Part model, mm, in its own coordinate system. Face numbers are marked on the shaded views. A direction names the side the tool comes from. Give positions to 0.01 mm unless a question says otherwise; leave off trailing zeros. Order: outer loops, then holes, each group sorted by start corner. A loop starts at its lowest first (then second) coordinate and runs counter-clockwise, first axis right, second up. Notation, with made-up numbers: (70.5, 23) - (85.5, 23) arc R23 ccw to (85.5, 31) - close; hole circle Ø11 at (63.5, 36.5). An arc over 180 degrees is marked (long way). Use a Markdown table: item, result. Add a question column.
from build123d import *

# Parameters (mm, degrees)
CYLINDER003_R           = 1.5
CYLINDER003_DEPTH       = 10
CYLINDER003_PITCH_ANGLE = -90
CYLINDER002_R           = 1.5
CYLINDER002_DEPTH       = 8
CYLINDER_R              = 1.5
CYLINDER_DEPTH          = 10
CYLINDER_PITCH_ANGLE    = -90
CYLINDER001_R           = 2
CYLINDER001_DEPTH       = 8
SKETCH_R                = 3
PAD_DEPTH               = 10


with BuildPart() as cilindro003:
    # Cylinder003 → Cylinder003 (new body)
    with BuildSketch(Plane.XY):
        Circle(CYLINDER003_R)
    extrude(amount=CYLINDER003_DEPTH)


with BuildPart() as cilindro003_1:
    # Cylinder003 pitch: moved
    add(cilindro003.part.rotate(Axis((0, 0, 0), (0, 1, 0)), CYLINDER003_PITCH_ANGLE))


with BuildPart() as cilindro003_2:
    # Cylinder003 placement: moved
    add(cilindro003_1.part.moved(Location((0.071563, 0, 7.897581))))


with BuildPart() as cilindro002:
    # Cylinder002 → Cylinder002 (new body)
    with BuildSketch(Plane.XY.offset(5)):
        Circle(CYLINDER002_R)
    extrude(amount=CYLINDER002_DEPTH)


with BuildPart() as cilindro:
    # Cylinder → Cylinder (new body)
    with BuildSketch(Plane.XY):
        Circle(CYLINDER_R)
    extrude(amount=CYLINDER_DEPTH)


with BuildPart() as cilindro_1:
    # Cylinder pitch: moved
    add(cilindro.part.rotate(Axis((0, 0, 0), (0, 1, 0)), CYLINDER_PITCH_ANGLE))


with BuildPart() as cilindro_2:
    # Cylinder placement: moved
    add(cilindro_1.part.moved(Location((1.071563, 0, 1.897581))))


with BuildPart() as cilindro001:
    # Cylinder001 → Cylinder001 (new body)
    with BuildSketch(Plane.XY.offset(-3)):
        Circle(CYLINDER001_R)
    extrude(amount=CYLINDER001_DEPTH)


with BuildPart() as cut003:
    # Sketch → Pad (new body)
    with BuildSketch(Plane.XY):
        Circle(SKETCH_R)
    extrude(amount=PAD_DEPTH)

    # Cut: cut Cilindro001
    add(cilindro001.part, mode=Mode.SUBTRACT)

    # Cut001: cut Cilindro
    add(cilindro_2.part, mode=Mode.SUBTRACT)

    # Cut002: cut Cilindro002
    add(cilindro002.part, mode=Mode.SUBTRACT)

    # Cut003: cut Cilindro003
    add(cilindro003_2.part, mode=Mode.SUBTRACT)


solid = cut003.part
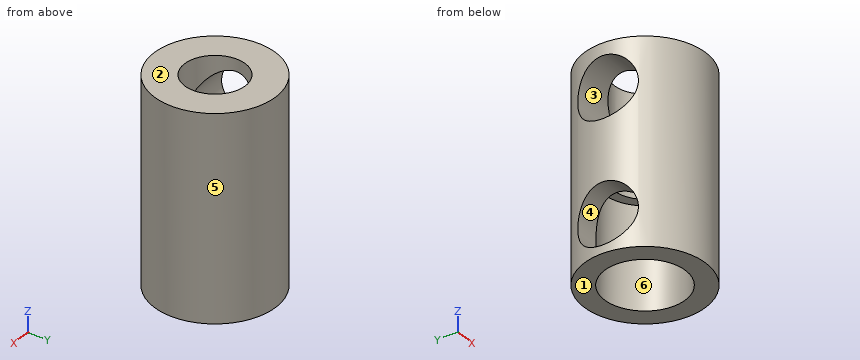
1. Drill centre lines: probe 1 along Y at (x, z) = (0, 3.8); probe 2 along Y at (x, z) = (0, 6.1); probe 3 along X at (y, z) = (0, 1.15). Where is each one in solid material? Low to high. Write a range as [from, to].
2. Cut at C-C (x = -1.75). Write the cut outline in (y, z), plus the area to 3 significant figures.
3. Pin check, flat tips, straight feed: P1, Ø1, axis at x = 1.5, y = 1.5, coming from the -Z side; P2, Ø1.5, axis at y = 1.5, z = 2.5, coming from the -X side; P3, Ø2, axis at x = -0.5, y = 0.5, coming from the -Z side. Stop position of each tip, or through.
4. Cut at B-B (x = -0.75). Write the cut outline in (y, z).
5. Tool access for the marked faces 4, 5 and 6: list every direction of +Z, -Z, +X, -X, +Y, -Y with a clear straight run to the whole face (end or side of a thin tool).
6. Cut at A-A (y = 0). Write the cut outline in (x, z).
7. Cut at D-D (y = -1). Write the cut outline in (x, z).
8. Mould opens along Z. For the marked faces 1, 2 and 3 say: released by +Z, released by -Z, zero draft, split by the parting line, or undercut.
Responses:
| question | item | result |
|---|---|---|
| 1 | probe 1 | y = [-3, -2], [2, 3] |
| 1 | probe 2 | y = [-3, -1.5], [1.5, 3] |
| 1 | probe 3 | x = [2, 3] |
| 2 | outline | (-2.44, 0) - (-0.97, 0) - (-0.97, 0.75) arc R1.5 cw to (-0.97, 3.04) - (-0.97, 5) - (0.97, 5) - (0.97, 3.04) arc R1.5 cw to (0.97, 0.75) - (0.97, 0) - (2.44, 0) - (2.44, 10) - (-2.44, 10) - close; hole circle Ø3 at (0, 7.9) |
| 2 | area | 30.3 mm² |
| 3 | P1 | stops at z = 0 |
| 3 | P2 | stops at x = -2.84 |
| 3 | P3 | stops at z = 5 |
| 4 | outline | (-2.9, 0) - (-1.85, 0) - (-1.85, 5) - (-1.3, 5) - (-1.3, 7.15) arc R1.5 cw to (-1.3, 8.65) - (-1.3, 10) - (-2.9, 10) - close; (1.3, 5) - (1.85, 5) - (1.85, 0) - (2.9, 0) - (2.9, 10) - (1.3, 10) - (1.3, 8.65) arc R1.5 cw to (1.3, 7.15) - close |
| 5 | face 4 | -X |
| 5 | face 5 | +Z, -Z |
| 5 | face 6 | -Z |
| 6 | outline | (-3, 0) - (-2, 0) - (-2, 0.4) - (-3, 0.4) - close; (-3, 3.4) - (-2, 3.4) - (-2, 5) - (-1.5, 5) - (-1.5, 6.4) - (-3, 6.4) - close; (-3, 9.4) - (-1.5, 9.4) - (-1.5, 10) - (-3, 10) - close; (1.5, 5) - (2, 5) - (2, 0) - (3, 0) - (3, 10) - (1.5, 10) - close |
| 7 | outline | (-2.83, 0) - (-1.73, 0) - (-1.73, 0.78) - (-2.83, 0.78) - close; (-2.83, 3.02) - (-1.73, 3.02) - (-1.73, 5) - (-1.12, 5) - (-1.12, 6.78) - (-2.83, 6.78) - close; (-2.83, 9.02) - (-1.12, 9.02) - (-1.12, 10) - (-2.83, 10) - close; (1.12, 5) - (1.73, 5) - (1.73, 0) - (2.83, 0) - (2.83, 10) - (1.12, 10) - close |
| 8 | face 1 | released by -Z |
| 8 | face 2 | released by +Z |
| 8 | face 3 | undercut |
